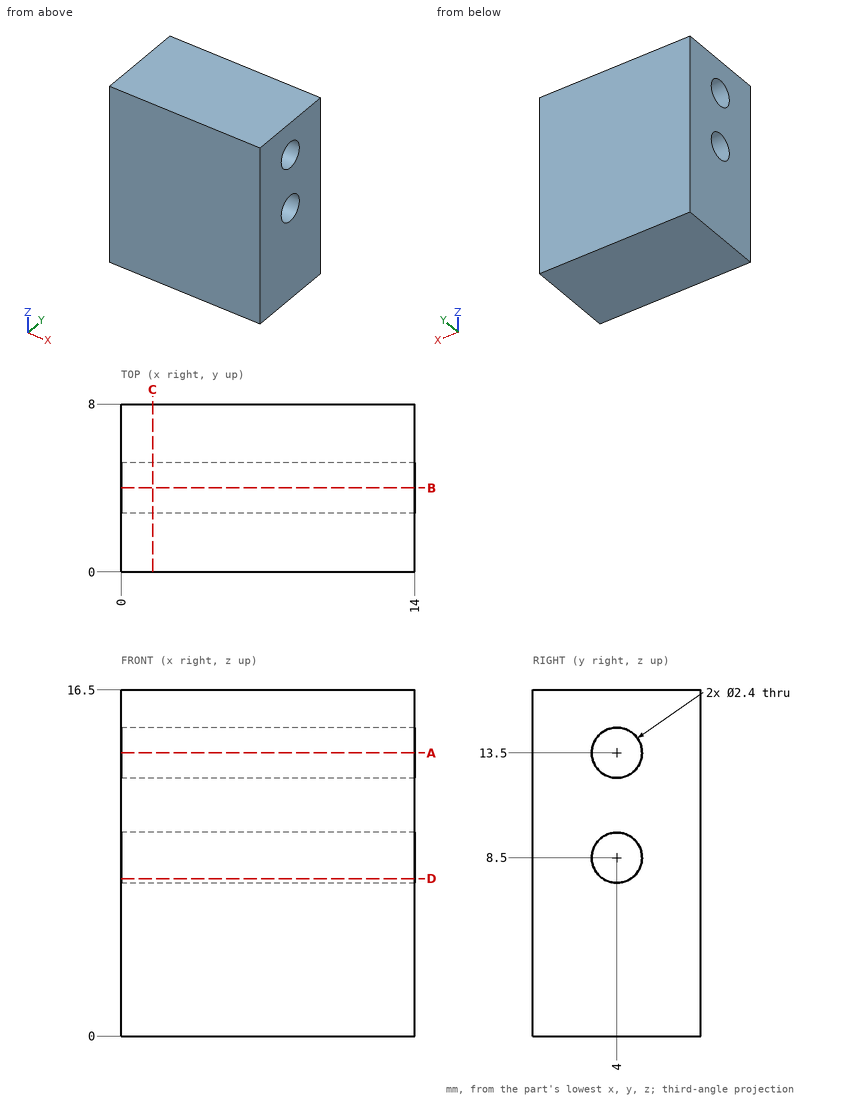
Here's the drawing with two shaded views (mm, measured from the low corner). I have some questions. Round coordinates to 2 decimals unless told otherwise and drop trailing zeros. Order: outer loops, then holes, each group sorted by start corner. A loop starts at its lowest first (then second) coordinate and runs counter-clockwise, first axis right, second up. Notation, with made-up numbers: (-36.5, -7) -> (-30.5, -7) arc R14 cw to (-30.5, 5) -> close; hole circle Ø8 at (14, 5). An arc over 180 degrees is marked (long way). Return JSON: item names as keys, results as strings.
Q1. If we section it at B-B on y = 4: List the corners of the cut face in (x, z) for me.
Filled sheet:
{"outline": "(0, 0) -> (14, 0) -> (14, 7.3) -> (0, 7.3) -> close; (0, 9.7) -> (14, 9.7) -> (14, 12.3) -> (0, 12.3) -> close; (0, 14.7) -> (14, 14.7) -> (14, 16.5) -> (0, 16.5) -> close"}
Q2. If we section it at C-C on x = 1.5: List the corners of the cut face in (y, z) for me.
Filled sheet:
{"outline": "(0, 0) -> (8, 0) -> (8, 16.5) -> (0, 16.5) -> close; hole circle Ø2.4 at (4, 8.5); hole circle Ø2.4 at (4, 13.5)"}
Q3. I need wall thicknesses on line 1 along Z through (x, y) = (7.75, 4); line 2 along Y through (x, z) = (9.5, 8.5); line 3 along Z through (x, y) = (5, 4.5). Which ranges of each line are inside material? Lowest first, please. Write a range as from..to.
Filled sheet:
{"line 1": "z = 0..7.3, 9.7..12.3, 14.7..16.5", "line 2": "y = 0..2.8, 5.2..8", "line 3": "z = 0..7.41, 9.59..12.41, 14.59..16.5"}
Q4. If we section it at D-D on z = 7.5: List the corners of the cut face in (x, y) for me.
Filled sheet:
{"outline": "(0, 0) -> (14, 0) -> (14, 3.34) -> (0, 3.34) -> close; (0, 4.66) -> (14, 4.66) -> (14, 8) -> (0, 8) -> close"}
Q5. If we section it at A-A on z = 13.5: List the corners of the cut face in (x, y) for me, plus the area to 3 significant figures.
Filled sheet:
{"outline": "(0, 0) -> (14, 0) -> (14, 2.8) -> (0, 2.8) -> close; (0, 5.2) -> (14, 5.2) -> (14, 8) -> (0, 8) -> close", "area": "78.4 mm^2"}
